```python
from build123d import *

# Parameters (mm, degrees)
F1_DEPTH = 25
F3_DEPTH = 10
F4_R     = 5.5
F5_DEPTH = 10
F6_R     = 2
F7_R     = 2


with BuildPart() as f1:
    # F0 (on Front) → F1 (new body)
    with BuildSketch(Plane.XZ):
        Polygon((10, 48), (0, 48), (0, 0), (-34, 0), (-34, -10), (10, -10), align=None)
    extrude(amount=F1_DEPTH)

    # F2 (on face) → F3 (cut)
    with BuildSketch(Plane(origin=(0, 0, -10), x_dir=(1, 0, 0), z_dir=(0, 0, -1))):
        with BuildLine():
            Line((-12.25, 16.75), (-25.75, 16.75))
            ThreePointArc((-25.75, 16.75), (-30, 12.5), (-25.75, 8.25))
            Line((-25.75, 8.25), (-12.25, 8.25))
            ThreePointArc((-12.25, 8.25), (-8, 12.5), (-12.25, 16.75))
        make_face()
    extrude(amount=-F3_DEPTH, mode=Mode.SUBTRACT)

    # F4 (on face) → F5 (cut)
    with BuildSketch(Plane.YZ.offset(10)):
        with Locations((-12.5, 13.5)):
            Circle(F4_R)
        with Locations((-12.5, 39)):
            Circle(F4_R)
    extrude(amount=-F5_DEPTH, mode=Mode.SUBTRACT)

    # F6
    f6_edges = [f1.edges().sort_by_distance(p)[0] for p in [
        (0, -12.5, 0),
    ]]
    fillet(f6_edges, radius=F6_R)

    # F7
    f7_edges = [f1.edges().sort_by_distance(p)[0] for p in [
        (10, -12.5, -10),
    ]]
    fillet(f7_edges, radius=F7_R)


solid = f1.part
```
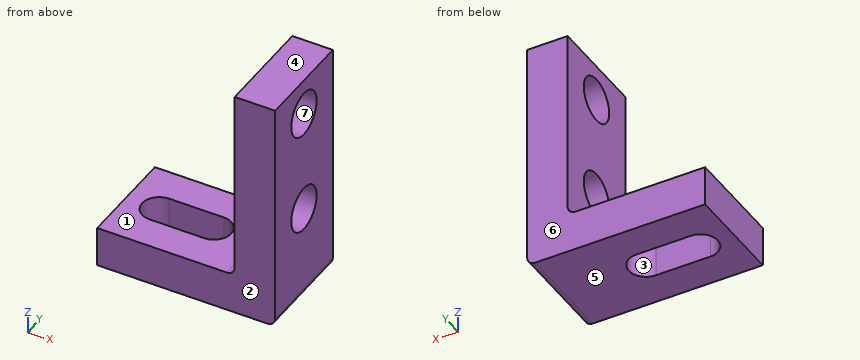
Input: part model. Units: mm. Frame: model coordinates. Face numbers are marked on the shaded views. A direction names the side the tool comes from. Round coordinates to 2 decimals unless told otherwise and drop trailing zeros. Loops run counter-clockwise (first coordinate to the right, second up) from the corner with the lowest first, then second, coordinate; pieces in that order, holes last. Notation, with made-up numbers: (32.25, 21) -> (53.25, 21) arc R34 cw to (53.25, 60) -> close; hole circle Ø11 at (-14.75, -9). An arc over 180 degrees is marked (long way). Write each question's results on one line, items separated by ' | '.
1. Section D-D (x = -9.5). Return loops of the section in (y, z), and give its area (3 significant figures).
Geometry results:
outline: (-25, -10) -> (-15.74, -10) -> (-15.74, 0) -> (-25, 0) -> close; (-9.26, -10) -> (0, -10) -> (0, 0) -> (-9.26, 0) -> close | area: 185 mm2
2. Section C-C (y = -11). Return loops of the section in (x, z), and give its area (3 significant figures).
Geometry results:
outline: (-34, -10) -> (-29.73, -10) -> (-29.73, 0) -> (-34, 0) -> close; (-8.27, -10) -> (8, -10) arc R2 ccw to (10, -8) -> (10, 8.21) -> (0, 8.21) -> (0, 2) arc R2 cw to (-2, 0) -> (-8.27, 0) -> close; (0, 18.79) -> (10, 18.79) -> (10, 33.71) -> (0, 33.71) -> close; (0, 44.29) -> (10, 44.29) -> (10, 48) -> (0, 48) -> close | area: 494 mm2
3. Section B-B (z = -5.5). Return loops of the section in (x, y), and give its area (3 significant figures).
Geometry results:
outline: (-34, -25) -> (10, -25) -> (10, 0) -> (-34, 0) -> close; hole (-25.75, -16.75) -> (-12.25, -16.75) arc R4.25 ccw to (-12.25, -8.25) -> (-25.75, -8.25) arc R4.25 ccw to start | area: 929 mm2
4. Ray query, line 1 (Z direction, x = 2.75, y = -12.5); line 2 (Z direction, x = 3, y = -14); line 3 (X direction, y = -6.5, z = 14). Return the intervals inside material, ascending. Write a range as from..to.
Geometry results:
line 1: -10..8, 19..33.5, 44.5..48 | line 2: -10..8.21, 18.79..33.71, 44.29..48 | line 3: 0..10
5. First-contact query: P1, Ø2, axis at y = -11, z = 26.5, coming from the -X side; P2, Ø4, axis at x = -15, y = -4.5, coming from the +Z side. Flat tips, straight axial feed; report the tip coordinate or a pass-through.
Geometry results:
P1: x = 0 | P2: z = 0
6. Mould query, pull axis Z, two halves, no side actions, for the marked faces 4, 5, 6 and 7. Classes: +Z half, -Z half, draft (parallel to the pull), parting line (faces both ways), or undercut.
Geometry results:
face 4: +Z half | face 5: -Z half | face 6: draft | face 7: undercut
7. Set-up query: the marked faces 1, 2 and 3. Return all of +Z, -Z, +X, -X, +Y, -Y with unobstructed straight access to the full face (end or side cutting, diameter ignored); none if empty.
Geometry results:
face 1: +Z, -X, +Y, -Y | face 2: +Z, -Z, +X, -X, -Y | face 3: +Z, -Z
8. Section A-A (z = 39). Return loops of the section in (x, y).
Geometry results:
outline: (0, -25) -> (10, -25) -> (10, -18) -> (0, -18) -> close; (0, -7) -> (10, -7) -> (10, 0) -> (0, 0) -> close
